Design review of the part shown in the three views and the two pictorial views. Dimensions are in mm from the part's minimum x, y and z. Coordinates: 2 decimals unless noted, no trailing zeros. Write each loop counter-clockwise with the first axis right and the second up, starting at its lowest first coordinate (ties: lowest second). Pieces come first, ordered by that corner, then holes. Notation, with made-up numbers: (73, 57) - (112, 57) arc R31 ccw to (112, 82) - close; hole circle Ø1 at (-18.5, 4.5). An arc over 180 degrees is marked (long way). Return JSON: item names as keys, results as strings. Group by question number.
(1) We need section D-D on z = 33. State the section outline as (x, y) points.
(2) We need section C-C on x = 4.25. State the section outline as (y, z) points, then the cut area to 3 significant figures.
(3) To check wall thickness, follow L1, parallel to Z at x = 0.45, y = 20; L2, parallel to X at y = 17.5, z = 6; L3, parallel to Y at x = 5.2, z = 20. State the ranges of each line that lie inside material, in increasing order. Write a range as from..to.
(4) Draft analysis for pull direction Y (two halves, no side actions). For the marked faces 1, 2 and 3, state which applies: released by +Y, released by -Y, zero draft, split by the parting line, or undercut.
(5) For pin 1 Ø3 at (y, z) = (22, 17.5) entering from -X; pin 2 Ø2.5 at (y, z) = (20, 20) entering from +X; pin 3 Ø8 at (y, z) = (26.5, 34.5) entering from -X; pin 4 Ø4 at (y, z) = (23, 20) entering from +X, all flat-tipped, find the tip position at first contact; note any pin that passes through.
(6) We need section A-A on y = 20. State the section outline as (x, z) points, then the cut area to 3 significant figures.
(7) We need section B-B on z = 20. State the section outline as (x, y) points.
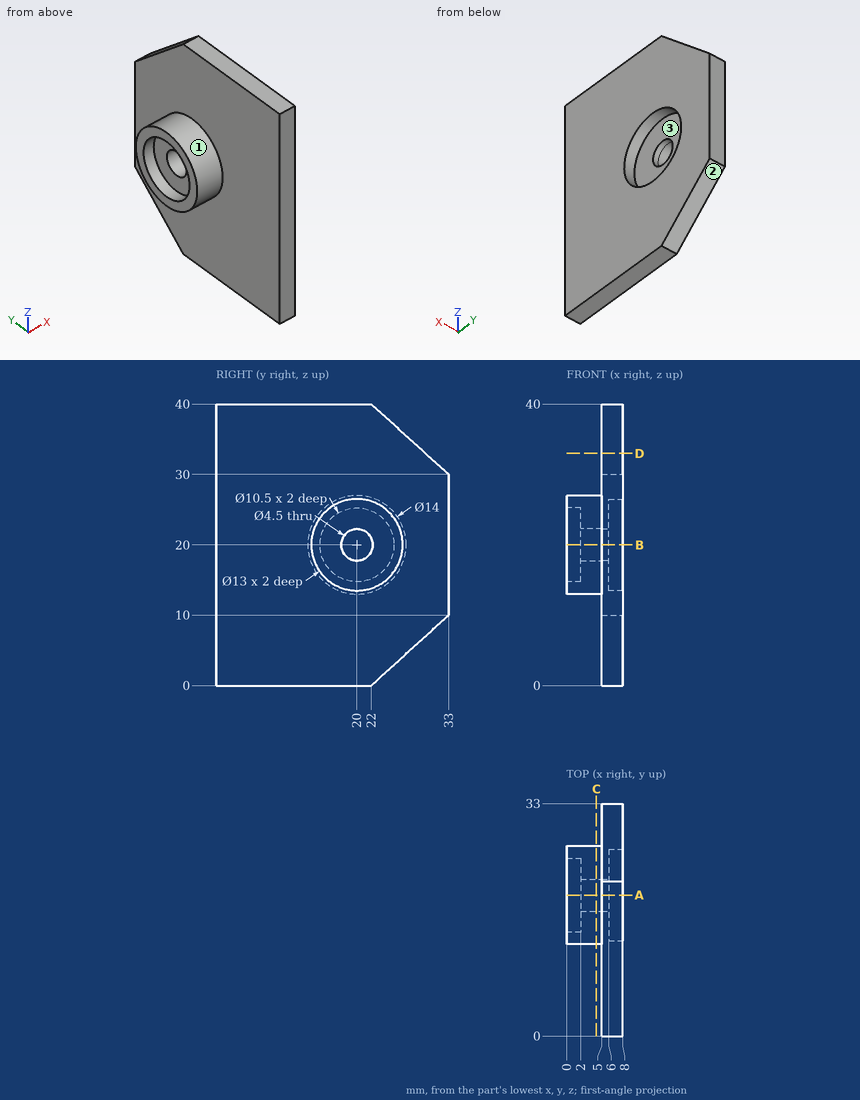
Ans:
{
 "1": {"outline": "(5, 0) - (8, 0) - (8, 29.7) - (5, 29.7) - close"},
 "2": {"outline": "circle Ø14 at (20, 20); hole circle Ø4.5 at (20, 20)", "area": "138 mm²"},
 "3": {"L1": "13..14.75, 25.25..27", "L2": "5..8", "L3": "0..17.75, 22.25..33"},
 "4": {"face 1": "split by the parting line", "face 2": "released by +Y", "face 3": "undercut"},
 "5": {"pin 1": "x = 2", "pin 2": "through", "pin 3": "x = 5", "pin 4": "x = 6"},
 "6": {"outline": "(0, 13) - (5, 13) - (5, 0) - (8, 0) - (8, 13.5) - (6, 13.5) - (6, 17.75) - (2, 17.75) - (2, 14.75) - (0, 14.75) - close; (0, 25.25) - (2, 25.25) - (2, 22.25) - (6, 22.25) - (6, 26.5) - (8, 26.5) - (8, 40) - (5, 40) - (5, 27) - (0, 27) - close", "area": "125 mm²"},
 "7": {"outline": "(0, 13) - (5, 13) - (5, 0) - (8, 0) - (8, 13.5) - (6, 13.5) - (6, 17.75) - (2, 17.75) - (2, 14.75) - (0, 14.75) - close; (0, 25.25) - (2, 25.25) - (2, 22.25) - (6, 22.25) - (6, 26.5) - (8, 26.5) - (8, 33) - (5, 33) - (5, 27) - (0, 27) - close"}
}
